```python
from build123d import *

# Parameters (mm, degrees)
SKETCH1_W           = 49.5
SKETCH1_H           = 61
SKETCH1_R           = 17.5
BOSS_EXTRUDE1_DEPTH = 8
FILLET1_R           = 2
SKETCH25_R          = 4.05
CUT_EXTRUDE24_DEPTH = 20


with BuildPart() as part:
    # Sketch1 → Boss-Extrude1 (new body)
    with BuildSketch(Plane.XY):
        with Locations((-375.83204095, -9.5)):
            Rectangle(SKETCH1_W, SKETCH1_H)
        with Locations((-375.83204095, -9.5)):
            Circle(SKETCH1_R, mode=Mode.SUBTRACT)
    extrude(amount=BOSS_EXTRUDE1_DEPTH)

    # Fillet1
    fillet1_edges = [part.edges().sort_by_distance(p)[0] for p in [
        (-400.58204095, -40, 4),
        (-400.58204095, 21, 4),
        (-351.08204095, 21, 4),
        (-351.08204095, -40, 4),
    ]]
    fillet(fillet1_edges, radius=FILLET1_R)

    # Sketch25 → Cut-Extrude24 (cut)
    with BuildSketch(Plane(origin=(-362.113949842, -45.191927803, 10), x_dir=(1, 0, 0), z_dir=(0, 0, 1))):
        with Locations((-30.468091108, 11.191927803)):
            Circle(SKETCH25_R)
        with Locations((-30.468091108, 60.191927803)):
            Circle(SKETCH25_R)
        with Locations((3.031908892, 11.191927803)):
            Circle(SKETCH25_R)
        with Locations((3.031908892, 60.191927803)):
            Circle(SKETCH25_R)
    extrude(amount=-CUT_EXTRUDE24_DEPTH, mode=Mode.SUBTRACT)


solid = part.part
```
CAD build for the part. Positions are in the model's coordinates, mm. Round coordinates to 2 decimals unless told otherwise and drop trailing zeros. Order: outer loops, then holes, each group sorted by start corner. A loop starts at its lowest first (then second) coordinate and runs counter-clockwise, first axis right, second up. Notation, with made-up numbers: (-2, -21) - (51, -21) arc R23 ccw to (51, -9) - close; hole circle Ø7 at (-1, -30.5). An arc over 180 degrees is marked (long way). Answer as CSV lines item,"result". Start each with the question number.
1. Saw through at B-B, the plane z = 3.75. Write the cut outline in (x, y).
2. Saw through at D-D, the plane y = -9.5. Write the cut outline in (x, z).
3. Saw through at A-A, the plane y = 15. Write the cut outline in (x, z), and give its area (3 significant figures).
4. Saw through at C-C, the plane x = -396. Write the cut outline in (y, z).
5. Pull direction X, two halves, no side cores. Call faces 1 (the face through (-400.01, -39.4, 4.06)), 2 (the face through (-387.2, 4.5, 0)), 3 (the face through (-351.082, -10, 4)), 4 (the face through (-355.22, -32.78, 4.06)): +X half, -X half, draft (parallel to the pull), parting line (faces both ways), or undercut.
6. Drill centre lines: L1, parallel to Y at x = -391, z = 1.75; L2, parallel to Y at x = -392, z = 1.25; L3, parallel to Y at x = -373, z = 3.5. Where is each one in solid material? Low to high. Write a range as [from, to].
7. Pin check, flat tip, straight feed: pin 1 (6 mm diameter, centred on x = -382.5, y = -21, fed in from -Z). Stop position of the tip, or through.
Model answer:
1,outline,"(-400.58, -38) arc R2 ccw to (-398.58, -40) - (-353.08, -40) arc R2 ccw to (-351.08, -38) - (-351.08, 19) arc R2 ccw to (-353.08, 21) - (-398.58, 21) arc R2 ccw to (-400.58, 19) - close; hole circle Ø8.1 at (-392.58, -34); hole circle Ø8.1 at (-392.58, 15); hole circle Ø35 at (-375.83, -9.5); hole circle Ø8.1 at (-359.08, -34); hole circle Ø8.1 at (-359.08, 15)"
2,outline,"(-400.58, 0) - (-393.33, 0) - (-393.33, 8) - (-400.58, 8) - close; (-358.33, 0) - (-351.08, 0) - (-351.08, 8) - (-358.33, 8) - close"
3,outline,"(-400.58, 0) - (-396.63, 0) - (-396.63, 8) - (-400.58, 8) - close; (-388.53, 0) - (-363.13, 0) - (-363.13, 8) - (-388.53, 8) - close; (-355.03, 0) - (-351.08, 0) - (-351.08, 8) - (-355.03, 8) - close"
3,area,"266 mm²"
4,outline,"(-40, 0) - (-36.17, 0) - (-36.17, 8) - (-40, 8) - close; (-31.83, 0) - (12.83, 0) - (12.83, 8) - (-31.83, 8) - close; (17.17, 0) - (21, 0) - (21, 8) - (17.17, 8) - close"
5,face 1,"-X half"
5,face 2,"draft"
5,face 3,"+X half"
5,face 4,"undercut"
6,L1,"y = [-40, -37.73], [-30.27, -18.23], [-0.77, 11.27], [18.73, 21]"
6,L2,"y = [-40, -38.01], [-29.99, -16.2], [-2.8, 10.99], [19.01, 21]"
6,L3,"y = [-40, -26.77], [7.77, 21]"
7,pin 1,"passes through"
